Here's how the part is built. I have some questions about the finished solid (model axes, mm). A direction names the side the tool comes from. Give positions to 0.01 mm unless a question says otherwise; leave off trailing zeros. Loops run counter-clockwise (first coordinate to the right, second up) from the corner with the lowest first, then second, coordinate; pieces in that order, holes last. Notation, with made-up numbers: (56.25, 52.25) - (82.25, 52.25) arc R7 cw to (82.25, 61.25) - close; hole circle Ø3 at (8, 77). An arc over 180 degrees is marked (long way). Return JSON: item names as keys, results as strings. Group by question number.
(1) For P1, Ø19.5, axis at x = -38, z = 23, coming from the +Y side; P2, Ø10.5, axis at y = 15.5, z = 7, coming from the -X side; P3, Ø25, axis at x = -41.21, z = 24.44, coming from the +Y side (3 decimals), each with a flat end and sliding along its axis, tell me the tip position at first contact or that it passes through.
(2) If we mould it in two halves opening along X, with no side actions, what happens to faces 1 (the flat face through (-41, 16.51, -2)), 2 (the flat face through (-42, 9.525, 9)), 3 (the flat face through (-41, -31.115, -2)), 4 (the flat face through (-18.987, 14, -1))? For each: released by +X, released by -X, zero draft, split by the parting line, or undercut.
(3) If we section it at A-A (z = 0): Please give me the cut outline in (x, y) (3 decimals).
(4) If we section it at D-D (x = 42.5): Please give me the cut outline in (y, z), then the cut area to 3 significant figures.
(5) I need wall thicknesses on probe 1 along Y at (x, z) = (-23, -16) (3 decimals); probe 2 along X at (y, z) = (-29.5, 25.5); probe 3 along X at (y, z) = (15, 0). Which ranges of each line are inside material? Lowest first, please. Write a range as [from, to].
(6) On a 3-axis mill with a long thin cutter (end or side, diameter ignored), from which of +Z, -Z, +X, -X, +Y, -Y can I reach the whole of each face in a straight line? I mean faces 5 (the flat face through (-42, -38.1, 1)), 6 (the flat face through (-63.437, 14, -1)), 7 (the cylindrical face through (-53.326, 17.798, 28.254)), 8 (the flat face through (-18.987, -33, -1)). Say none if no direction works.
(7) If we section it at C-C (z = -46): Please give me the cut outline in (x, y), then the cut area to 3 significant figures.
(8) If we section it at B-B (y = -16): Please give me the cut outline in (x, z).
```python
from build123d import *

# Parameters (mm, degrees)
F0_W            = 304.8
F0_H            = 35.6965847313
F1_DEPTH        = 63.5
F2_W            = 25.4
F2_H            = 44.45
F3_DEPTH        = 152.4
F4_W            = 44.45
F4_H            = 9.525
F5_DEPTH        = 57.15
F6_DEPTH        = 57.15
F9_DEPTH        = 9.525
F10_DEPTH       = 9.525
F11_W           = 304.8
F11_H           = 114.3
F12_DEPTH       = 31.75
F13_T           = -2.54
F16_D           = 19.05
F16_DEPTH       = 9.525
F16_CBORE_D     = 25.4
F16_CBORE_DEPTH = 3.81
F16_TIP         = 5.7231973962
F17_D           = 19.05
F17_DEPTH       = 9.525
F17_CBORE_D     = 25.4
F17_CBORE_DEPTH = 3.81
F17_TIP         = 5.7231973962


with BuildPart() as f1:
    # F0 (on Front) → F1 (new body, symmetric)
    with BuildSketch(Plane.XZ):
        with Locations((25.4629384518, -47.1194889396)):
            Rectangle(F0_W, F0_H)
    extrude(amount=F1_DEPTH, both=True)

    # F2 (on face) → F3 (cut)
    with BuildSketch(Plane.XZ.offset(63.5)):
        with BuildLine():
            ThreePointArc((-37.1512658894, 15.178803426), (-49.8512658894, 27.878803426), (-62.5512658894, 15.178803426))
            Line((-62.5512658894, 15.178803426), (-37.1512658894, 15.178803426))
        make_face()
        with Locations((-49.8512658894, -7.046196574)):
            Rectangle(F2_W, F2_H)
    extrude(amount=-F3_DEPTH, mode=Mode.SUBTRACT)

    # F4 (on face) → F5 (join)
    with BuildSketch(Plane.XY.offset(-29.271196574)):
        with Locations((-41.2120615482, 14.2875)):
            Rectangle(F4_W, F4_H)
    extrude(amount=F5_DEPTH)

    # F4 (on face) → F6 (join)
    with BuildSketch(Plane.XY.offset(-29.271196574)):
        with Locations((-41.2120615482, 14.2875)):
            Rectangle(F4_W, F4_H)
        with Locations((-41.2120615482, -33.3375)):
            Rectangle(F4_W, F4_H)
    extrude(amount=F6_DEPTH)

    # F7 (on face) → F9 (join)
    with BuildSketch(Plane.XZ.offset(38.1)):
        with BuildLine():
            Line((-63.4370615482, 27.878803426), (-18.9870615482, 27.878803426))
            ThreePointArc((-18.9870615482, 27.878803426), (-41.2120615482, 46.928803426), (-63.4370615482, 27.878803426))
        make_face()
    extrude(amount=-F9_DEPTH)

    # F8 (on face) → F10 (join)
    with BuildSketch(Plane.XZ.offset(-9.525)):
        with BuildLine():
            Line((-63.4370615482, 27.878803426), (-18.9870615482, 27.878803426))
            ThreePointArc((-18.9870615482, 27.878803426), (-41.2120615482, 46.928803426), (-63.4370615482, 27.878803426))
        make_face()
    extrude(amount=-F10_DEPTH)

    # F11 (on face) → F12 (join)
    with BuildSketch(Plane(origin=(0, 0, -64.9677813053), x_dir=(1, 0, 0), z_dir=(0, 0, -1))):
        with Locations((25.4629384518, 0.6365377843)):
            Rectangle(F11_W, F11_H)
    extrude(amount=-F12_DEPTH)

    # F13
    f13_openings = [f1.faces().sort_by_distance(p)[0] for p in [
        (-126.937062, 0, -47.119489),
        (177.862938, 0, -47.119489),
    ]]
    offset(amount=F13_T, openings=f13_openings, kind=Kind.INTERSECTION)

    # F16
    with Locations(Plane.XZ.offset(38.1)):
        with Locations((-41.2120615482, 24.4392200927)):
            CounterBoreHole(F16_D / 2, F16_CBORE_D / 2, F16_CBORE_DEPTH, depth=F16_DEPTH)
            with Locations((0, 0, -(F16_DEPTH + F16_TIP / 2))):  # 118° drill point
                Cone(0, F16_D / 2, F16_TIP, mode=Mode.SUBTRACT)

    # F17
    with Locations(Plane(origin=(0, 19.05, 0), x_dir=(-1, 0, 0), z_dir=(0, 1, 0))):
        with Locations((41.2120615482, 24.4392200927)):
            CounterBoreHole(F17_D / 2, F17_CBORE_D / 2, F17_CBORE_DEPTH, depth=F17_DEPTH)
            with Locations((0, 0, -(F17_DEPTH + F17_TIP / 2))):  # 118° drill point
                Cone(0, F17_D / 2, F17_TIP, mode=Mode.SUBTRACT)


solid = f1.part
```
Values:
{
 "1": {"P1": "y = 19.05", "P2": "x = -63.44", "P3": "y = 12.065"},
 "2": {"face 1": "undercut", "face 2": "zero draft", "face 3": "undercut", "face 4": "released by +X"},
 "3": {"outline": "(-63.437, -38.1) - (-18.987, -38.1) - (-18.987, -28.575) - (-63.437, -28.575) - close; (-63.437, 9.525) - (-18.987, 9.525) - (-18.987, 19.05) - (-63.437, 19.05) - close; hole (-60.897, -35.56) - (-21.527, -35.56) - (-21.527, -31.115) - (-60.897, -31.115) - close; hole (-60.897, 12.065) - (-21.527, 12.065) - (-21.527, 16.51) - (-60.897, 16.51) - close"},
 "4": {"outline": "(-63.5, -64.97) - (63.5, -64.97) - (63.5, -29.27) - (-63.5, -29.27) - close; hole (-60.96, -62.43) - (60.96, -62.43) - (60.96, -31.81) - (-60.96, -31.81) - close", "area": "801 mm2"},
 "5": {"probe 1": "[-38.1, -35.56], [-31.115, -28.575], [9.525, 12.065], [16.51, 19.05]", "probe 2": "[-63.44, -50.68], [-31.75, -18.99]", "probe 3": "[-63.44, -60.9], [-21.53, -18.99]"},
 "6": {"face 5": "+Z, +X, -X, -Y", "face 6": "+Z, -X, +Y, -Y", "face 7": "+Y", "face 8": "+Z, +X, +Y, -Y"},
 "7": {"outline": "(-126.94, -63.5) - (177.86, -63.5) - (177.86, -60.96) - (-126.94, -60.96) - close; (-126.94, 60.96) - (177.86, 60.96) - (177.86, 63.5) - (-126.94, 63.5) - close", "area": "1,550 mm2"},
 "8": {"outline": "(-126.94, -64.97) - (177.86, -64.97) - (177.86, -62.43) - (-126.94, -62.43) - close; (-126.94, -31.81) - (177.86, -31.81) - (177.86, -29.27) - (-126.94, -29.27) - close"}
}
